For this review, take the finished solid that the model builds, in its own axes (mm). Face numbers are marked on the shaded views. A direction names the side the tool comes from. Round coordinates to 2 decimals unless told otherwise and drop trailing zeros. Order: outer loops, then holes, each group sorted by start corner. A loop starts at its lowest first (then second) coordinate and runs counter-clockwise, first axis right, second up. Notation, with made-up numbers: (21.25, 54) - (57.25, 54) arc R22 ccw to (57.25, 90) - close; hole circle Ø3 at (-26.5, 40.5). An arc over 180 degrees is marked (long way). One line per question, with ' | ' between items.
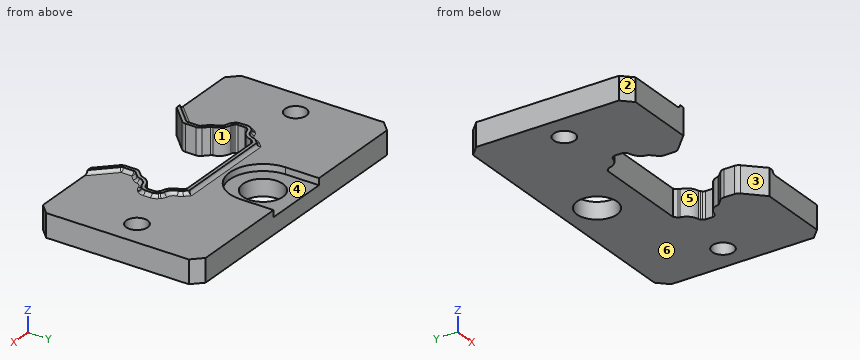
```python
from build123d import *

# Parameters (mm, degrees)
ENDSEAL_1_DEPTH              = 3.5
BOSS_EXTRUDE1_DEPTH          = 0.5
FILLET1_R                    = 0.5
F_6_0_6_DIAMETER_HOLE1_D     = 6
F_6_0_6_DIAMETER_HOLE1_DEPTH = 12.5
F_6_0_6_DIAMETER_HOLE1_TIP   = 1.561701152
CUT_EXTRUDE2_DEPTH           = 1
F_3_2_3_2_DIAMETER_HOLE1_D   = 3.2


with BuildPart() as part:
    # Sketch4 → Endseal 1 (new body)
    with BuildSketch(Plane.XY):
        with BuildLine():
            Line((-7.230720611, 12.9), (7.230720611, 12.9))
            Line((7.230720611, 12.9), (7.647672674, 12.483047938))
            ThreePointArc((7.647672674, 12.483047938), (7.736182466, 12.363118479), (7.785406885, 12.222427275))
            ThreePointArc((7.785406885, 12.222427275), (8.344607784, 11.164307384), (9.402727675, 10.605106485))
            ThreePointArc((9.402727675, 10.605106485), (9.54341888, 10.555882066), (9.663348338, 10.467372274))
            Line((9.663348338, 10.467372274), (9.853553391, 10.277167221))
            ThreePointArc((9.853553391, 10.277167221), (9.961939766, 10.114955546), (10, 9.92361383))
            Line((10, 9.92361383), (10, 8.86638617))
            ThreePointArc((10, 8.86638617), (9.961939766, 8.675044454), (9.853553391, 8.512832779))
            Line((9.853553391, 8.512832779), (9.675343394, 8.334622782))
            ThreePointArc((9.675343394, 8.334622782), (9.554347216, 8.245550888), (9.412352167, 8.19644607))
            ThreePointArc((9.412352167, 8.19644607), (8.344607784, 7.635448616), (7.783610331, 6.567704234))
            ThreePointArc((7.783610331, 6.567704234), (7.734505512, 6.425709184), (7.645433618, 6.304713007))
            Line((7.645433618, 6.304713007), (6.892893219, 5.552172608))
            ThreePointArc((6.892893219, 5.552172608), (6.676120468, 5.227749259), (6.6, 4.845065826))
            Line((6.6, 4.845065826), (6.6, 3.284934173))
            ThreePointArc((6.6, 3.284934173), (6.676120468, 2.902250741), (6.892893219, 2.577827392))
            Line((6.892893219, 2.577827392), (9.470720611, 0))
            Line((9.470720611, 0), (19.9998779, 0))
            Line((19.9998779, 0), (21.5, 1.5))
            Line((21.5, 1.5), (21.5, 22.9))
            Line((21.5, 22.9), (20.0001221, 24.4))
            Line((20.0001221, 24.4), (-19.9998779, 24.4))
            Line((-19.9998779, 24.4), (-21.5, 22.8997558))
            Line((-21.5, 22.8997558), (-21.5, 1.5))
            Line((-21.5, 1.5), (-19.9998779, 0))
            Line((-19.9998779, 0), (-9.470720611, 0))
            Line((-9.470720611, 0), (-6.892893219, 2.577827392))
            ThreePointArc((-6.892893219, 2.577827392), (-6.676120468, 2.902250741), (-6.6, 3.284934173))
            Line((-6.6, 3.284934173), (-6.6, 4.845065826))
            ThreePointArc((-6.6, 4.845065826), (-6.676120468, 5.227749259), (-6.892893219, 5.552172608))
            Line((-6.892893219, 5.552172608), (-7.645433618, 6.304713006))
            ThreePointArc((-7.645433618, 6.304713006), (-7.734505512, 6.425709184), (-7.783610331, 6.567704233))
            ThreePointArc((-7.783610331, 6.567704233), (-8.344607784, 7.635448616), (-9.412352167, 8.19644607))
            ThreePointArc((-9.412352167, 8.19644607), (-9.554347216, 8.245550888), (-9.675343394, 8.334622782))
            Line((-9.675343394, 8.334622782), (-9.853553391, 8.512832779))
            ThreePointArc((-9.853553391, 8.512832779), (-9.961939766, 8.675044454), (-10, 8.86638617))
            Line((-10, 8.86638617), (-10, 9.92361383))
            ThreePointArc((-10, 9.92361383), (-9.961939766, 10.114955546), (-9.853553391, 10.277167221))
            Line((-9.853553391, 10.277167221), (-9.663348338, 10.467372274))
            ThreePointArc((-9.663348338, 10.467372274), (-9.543418879, 10.555882066), (-9.402727675, 10.605106485))
            ThreePointArc((-9.402727675, 10.605106485), (-8.344607784, 11.164307384), (-7.785406885, 12.222427275))
            ThreePointArc((-7.785406885, 12.222427275), (-7.736182466, 12.363118479), (-7.647672674, 12.483047938))
            Line((-7.647672674, 12.483047938), (-7.230720611, 12.9))
        make_face()
    extrude(amount=ENDSEAL_1_DEPTH)

    # Sketch6 → Boss-Extrude1 (add)
    with BuildSketch(Plane.XY.offset(3.5)):
        with BuildLine():
            Line((-10.177827392, 0), (-7.24644661, 2.931380783))
            ThreePointArc((-7.24644661, 2.931380783), (-7.138060234, 3.093592457), (-7.1, 3.284934173))
            Line((-7.1, 3.284934173), (-7.1, 4.845065826))
            ThreePointArc((-7.1, 4.845065826), (-7.138060234, 5.036407542), (-7.24644661, 5.198619217))
            Line((-7.24644661, 5.198619217), (-7.998987008, 5.951159616))
            ThreePointArc((-7.998987008, 5.951159616), (-8.177130797, 6.193151971), (-8.275340434, 6.47714207))
            ThreePointArc((-8.275340434, 6.47714207), (-8.698161175, 7.281895225), (-9.50291433, 7.704715966))
            ThreePointArc((-9.50291433, 7.704715966), (-9.786904429, 7.802925603), (-10.028896784, 7.981069392))
            Line((-10.028896784, 7.981069392), (-10.207106781, 8.159279389))
            ThreePointArc((-10.207106781, 8.159279389), (-10.423879533, 8.483702737), (-10.5, 8.86638617))
            Line((-10.5, 8.86638617), (-10.5, 9.92361383))
            ThreePointArc((-10.5, 9.92361383), (-10.423879533, 10.306297262), (-10.207106781, 10.630720611))
            Line((-10.207106781, 10.630720611), (-10.016901728, 10.820925664))
            ThreePointArc((-10.016901728, 10.820925664), (-9.777042812, 10.99794525), (-9.495660403, 11.096394087))
            ThreePointArc((-9.495660403, 11.096394087), (-8.698161175, 11.517860775), (-8.276694487, 12.315360003))
            ThreePointArc((-8.276694487, 12.315360003), (-8.17824565, 12.596742412), (-8.001226064, 12.836601328))
            Line((-8.001226064, 12.836601328), (-7.437827392, 13.4))
            Line((-7.437827392, 13.4), (7.437827392, 13.4))
            Line((7.437827392, 13.4), (8.001226064, 12.836601328))
            ThreePointArc((8.001226064, 12.836601328), (8.17824565, 12.596742412), (8.276694487, 12.315360003))
            ThreePointArc((8.276694487, 12.315360003), (8.698161175, 11.517860775), (9.495660403, 11.096394087))
            ThreePointArc((9.495660403, 11.096394087), (9.777042812, 10.99794525), (10.016901728, 10.820925664))
            Line((10.016901728, 10.820925664), (10.207106781, 10.630720611))
            ThreePointArc((10.207106781, 10.630720611), (10.423879533, 10.306297262), (10.5, 9.92361383))
            Line((10.5, 9.92361383), (10.5, 8.86638617))
            ThreePointArc((10.5, 8.86638617), (10.423879533, 8.483702738), (10.207106781, 8.159279389))
            Line((10.207106781, 8.159279389), (10.028896784, 7.981069392))
            ThreePointArc((10.028896784, 7.981069392), (9.786904429, 7.802925604), (9.50291433, 7.704715966))
            ThreePointArc((9.50291433, 7.704715966), (8.698161175, 7.281895225), (8.275340434, 6.47714207))
            ThreePointArc((8.275340434, 6.47714207), (8.177130797, 6.193151971), (7.998987008, 5.951159616))
            Line((7.998987008, 5.951159616), (7.24644661, 5.198619217))
            ThreePointArc((7.24644661, 5.198619217), (7.138060234, 5.036407543), (7.1, 4.845065826))
            Line((7.1, 4.845065826), (7.1, 3.284934173))
            ThreePointArc((7.1, 3.284934173), (7.138060234, 3.093592457), (7.24644661, 2.931380783))
            Line((7.24644661, 2.931380783), (10.177827392, 0))
            Line((10.177827392, 0), (9.470720611, 0))
            Line((9.470720611, 0), (6.892893219, 2.577827392))
            ThreePointArc((6.892893219, 2.577827392), (6.676120468, 2.902250741), (6.6, 3.284934173))
            Line((6.6, 3.284934173), (6.6, 4.845065826))
            ThreePointArc((6.6, 4.845065826), (6.676120468, 5.227749259), (6.892893219, 5.552172608))
            Line((6.892893219, 5.552172608), (7.645433618, 6.304713007))
            ThreePointArc((7.645433618, 6.304713007), (7.734505512, 6.425709184), (7.783610331, 6.567704234))
            ThreePointArc((7.783610331, 6.567704234), (8.344607784, 7.635448616), (9.412352167, 8.19644607))
            ThreePointArc((9.412352167, 8.19644607), (9.554347216, 8.245550888), (9.675343394, 8.334622782))
            Line((9.675343394, 8.334622782), (9.853553391, 8.512832779))
            ThreePointArc((9.853553391, 8.512832779), (9.961939766, 8.675044454), (10, 8.86638617))
            Line((10, 8.86638617), (10, 9.92361383))
            ThreePointArc((10, 9.92361383), (9.961939766, 10.114955546), (9.853553391, 10.277167221))
            Line((9.853553391, 10.277167221), (9.663348338, 10.467372274))
            ThreePointArc((9.663348338, 10.467372274), (9.54341888, 10.555882066), (9.402727675, 10.605106485))
            ThreePointArc((9.402727675, 10.605106485), (8.344607784, 11.164307384), (7.785406885, 12.222427275))
            ThreePointArc((7.785406885, 12.222427275), (7.736182466, 12.363118479), (7.647672674, 12.483047938))
            Line((7.647672674, 12.483047938), (7.230720611, 12.9))
            Line((7.230720611, 12.9), (-7.230720611, 12.9))
            Line((-7.230720611, 12.9), (-7.647672674, 12.483047938))
            ThreePointArc((-7.647672674, 12.483047938), (-7.736182466, 12.363118479), (-7.785406885, 12.222427275))
            ThreePointArc((-7.785406885, 12.222427275), (-8.344607784, 11.164307384), (-9.402727675, 10.605106485))
            ThreePointArc((-9.402727675, 10.605106485), (-9.543418879, 10.555882066), (-9.663348338, 10.467372274))
            Line((-9.663348338, 10.467372274), (-9.853553391, 10.277167221))
            ThreePointArc((-9.853553391, 10.277167221), (-9.961939766, 10.114955546), (-10, 9.92361383))
            Line((-10, 9.92361383), (-10, 8.86638617))
            ThreePointArc((-10, 8.86638617), (-9.961939766, 8.675044454), (-9.853553391, 8.512832779))
            Line((-9.853553391, 8.512832779), (-9.675343394, 8.334622782))
            ThreePointArc((-9.675343394, 8.334622782), (-9.554347216, 8.245550888), (-9.412352167, 8.19644607))
            ThreePointArc((-9.412352167, 8.19644607), (-8.344607784, 7.635448616), (-7.783610331, 6.567704233))
            ThreePointArc((-7.783610331, 6.567704233), (-7.734505512, 6.425709184), (-7.645433618, 6.304713006))
            Line((-7.645433618, 6.304713006), (-6.892893219, 5.552172608))
            ThreePointArc((-6.892893219, 5.552172608), (-6.676120468, 5.227749259), (-6.6, 4.845065826))
            Line((-6.6, 4.845065826), (-6.6, 3.284934173))
            ThreePointArc((-6.6, 3.284934173), (-6.676120468, 2.902250741), (-6.892893219, 2.577827392))
            Line((-6.892893219, 2.577827392), (-9.470720611, 0))
            Line((-9.470720611, 0), (-10.177827392, 0))
        make_face()
    extrude(amount=BOSS_EXTRUDE1_DEPTH)

    # Fillet1
    fillet1_edges = [part.edges().sort_by_distance(p)[0] for p in [
        (-7.719526728, 13.118300664, 3.5),
        (-8.17824565, 12.596742412, 3.5),
        (-8.698161175, 11.517860775, 3.5),
        (-9.777042812, 10.99794525, 3.5),
        (-10.112004255, 10.725823138, 3.5),
        (-10.423879533, 10.306297262, 3.5),
        (-10.5, 9.395, 3.5),
        (-10.423879533, 8.483702737, 3.5),
        (-10.118001783, 8.07017439, 3.5),
        (-9.786904429, 7.802925603, 3.5),
        (-8.698161175, 7.281895225, 3.5),
        (-8.177130797, 6.193151971, 3.5),
        (-7.622716809, 5.574889416, 3.5),
        (-7.138060234, 5.036407542, 3.5),
        (-7.1, 4.065, 3.5),
        (-7.138060234, 3.093592457, 3.5),
        (7.719526728, 13.118300664, 3.5),
        (8.17824565, 12.596742412, 3.5),
        (8.698161175, 11.517860775, 3.5),
        (9.777042812, 10.99794525, 3.5),
        (10.112004255, 10.725823138, 3.5),
        (10.423879533, 10.306297262, 3.5),
        (10.5, 9.395, 3.5),
        (10.423879533, 8.483702738, 3.5),
        (10.118001783, 8.07017439, 3.5),
        (9.786904429, 7.802925604, 3.5),
        (8.698161175, 7.281895225, 3.5),
        (8.177130797, 6.193151971, 3.5),
        (7.622716809, 5.574889417, 3.5),
        (7.138060234, 5.036407543, 3.5),
        (7.1, 4.065, 3.5),
        (7.138060234, 3.093592457, 3.5),
        (-8.712137001, 1.465690391, 3.5),
        (0, 13.4, 3.5),
        (8.712137001, 1.465690391, 3.5),
    ]]
    fillet(fillet1_edges, radius=FILLET1_R - 0.0001)  # a hair under: the kernel refuses the full size

    # Ø6.0 (6) Diameter Hole1
    with Locations(Plane.XY.offset(3.5)):
        with Locations((0, 19.4)):
            Hole(F_6_0_6_DIAMETER_HOLE1_D / 2, depth=F_6_0_6_DIAMETER_HOLE1_DEPTH)
            with Locations((0, 0, -(F_6_0_6_DIAMETER_HOLE1_DEPTH + F_6_0_6_DIAMETER_HOLE1_TIP / 2))):  # 125° drill point
                Cone(0, F_6_0_6_DIAMETER_HOLE1_D / 2, F_6_0_6_DIAMETER_HOLE1_TIP, mode=Mode.SUBTRACT)

    # Sketch9 → Cut-Extrude2 (cut)
    with BuildSketch(Plane.XY.offset(3.5)):
        with BuildLine():
            Line((5, 19.4), (5, 35))
            Line((5, 35), (-5, 35))
            Line((-5, 35), (-5, 19.4))
            ThreePointArc((-5, 19.4), (0, 14.4), (5, 19.4))
        make_face()
    extrude(amount=-CUT_EXTRUDE2_DEPTH, mode=Mode.SUBTRACT)

    # Ø3.2 (3.2) Diameter Hole1 (through all)
    with Locations(Plane.XY.offset(3.5)):
        with Locations((-17.5, 12.4), (17.5, 12.4)):
            Hole(F_3_2_3_2_DIAMETER_HOLE1_D / 2)


solid = part.part
```
(1) Mouldability with a two-part tool opening along Z and no side actions: class the marked faces 4, 5 and 6 as released by +Z, released by -Z, zero draft, split by the parting line, or undercut.
Output values:
face 4: released by +Z | face 5: zero draft | face 6: released by -Z
(2) We need section C-C on z = 2. Give the number of separate pieces and of enclosed holes in the cut face, plus the area to 3 significant figures.
Output values:
separate pieces: 1 | enclosed holes: 3 | area: 792 mm^2
(3) For the marked faces 1, 2 and 3, list the 3-axis set-ups (+Z, -Z, +X, -X, +Y, -Y) from which the entire face can be reached by the end or side of a thin tool; tool diameter is ignored.
Output values:
face 1: +Z, -Z | face 2: +Z, -Z, -X, -Y | face 3: +Z, -Z, -Y
(4) Insertion check: pin 1 (2 mm diameter, centred on x = 1.5, z = 2.5, fed in from -Y); pin 2 (2 mm diameter, centred on x = 6.5, z = 2, fed in from -Y); pin 3 (9.5 mm diameter, centred on x = 0, y = 19.4, fed in from +Z). Each pin has a flat end and moves straight along its axis. Give the tip position at first contact, or say it passes through.
Output values:
pin 1: y = 12.9 | pin 2: y = 1.97 | pin 3: z = 2.5
(5) We need section A-A on x = 17.5. State the section outline as (y, z) points, plus the area to 3 significant figures.
Output values:
outline: (0, 0) - (10.8, 0) - (10.8, 3.5) - (0, 3.5) - close; (14, 0) - (24.4, 0) - (24.4, 3.5) - (14, 3.5) - close | area: 74.2 mm^2
(6) We need section B-B on y = 17.75. State the section outline as (x, z) points.
Output values:
outline: (-21.5, 0) - (-2.51, 0) - (-2.51, 2.5) - (-4.72, 2.5) - (-4.72, 3.5) - (-21.5, 3.5) - close; (2.51, 0) - (21.5, 0) - (21.5, 3.5) - (4.72, 3.5) - (4.72, 2.5) - (2.51, 2.5) - close
(7) For probe 1 along Y at (x, z) = (0, 1.85); probe 2 along X at (y, z) = (22.25, 2.95); probe 3 along Y at (x, z) = (17.5, 2.6), list the stretches that pass through material, from the lowest coordinate up. Write a range as [from, to].
Output values:
probe 1: [12.9, 16.4], [22.4, 24.4] | probe 2: [-21.5, -5], [5, 21.5] | probe 3: [0, 10.8], [14, 24.4]
